The listing builds one solid part. Answer for the finished solid, in the listing's coordinates (mm). Coordinates: 2 decimals unless noted, no trailing zeros. Loops run counter-clockwise (first coordinate to the right, second up) from the corner with the lowest first, then second, coordinate; pieces in that order, holes last. Notation, with made-up numbers: M 7,12 L 32,12 A28 cw 32,45 Z; hole C -1.5,40.25 d4. An arc over 180 degrees is marked long. Return JSON: item names as keys, results as strings. Group by question number.
1. Section A-A (z = -56.5) is taken. Write down the section's boundary in (x, y), then the cut area to 3 significant figures.
2. Section D-D (x = 64) is taken. Write down the section's boundary in (y, z).
3. Section B-B (y = 0.7) is taken. Count the separate pieces of the cut face and the enclosed holes in it, then the cut area to 3 significant figures.
4. Section C-C (z = 13) is taken. Write down the section's boundary in (x, y), then the cut area to 3 significant figures.
5. Given P1, Ø1.3, axis at y = 1, z = 66, coming from the +X side; P2, Ø1.2, axis at y = 1.5, z = 69, coming from the +X side; P3, Ø1.2, axis at y = 1, z = 69, coming from the -X side, each flat-ended and moving along its own axis, determine where each tip first touches the part or whether it passes through.
6. Straight lines are drawn through the part: L1, parallel to X at y = 2.4, z = -7; L2, parallel to X at y = 2.9, z = -66.5; L3, parallel to Z at x = -30, y = 2.5. For each, find the intervals that lie inside material, in ascending order. Write a range as from..to.
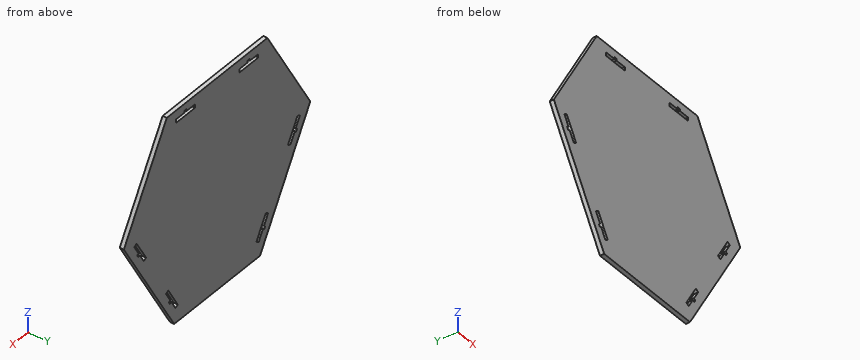
```python
from build123d import *

# Parameters (mm, degrees)
BOSS_EXTRUDE1_DEPTH      = 3
CUT_EXTRUDE1_DEPTH       = 119.131597452
CIRPATTERN1_COUNT        = 3
CIRPATTERN1_COPY_1_DEPTH = 119.131597452
CIRPATTERN1_COPY_2_DEPTH = 119.131597452


with BuildPart() as part:
    # Sketch1 → Boss-Extrude1 (new body)
    with BuildSketch(Plane(origin=(0, 0, 0), x_dir=(1, 0, 0), z_dir=(0, 1, 0))):
        Polygon((-40.640000094, 78.456128134), (40.639999906, 78.456128134), (88.265000282, -4.032791576), (47.624999812, -74.423336558), (-47.625, -74.423336558), (-88.265000094, -4.032791576), align=None)
    extrude(amount=BOSS_EXTRUDE1_DEPTH)

    # Sketch2 → Cut-Extrude1 (cut, through all)
    with BuildSketch(Plane(origin=(0, 3, 0), x_dir=(1, 0, 0), z_dir=(0, 1, 0))):
        Polygon((29, -68), (29, -69.5), (31, -69.5), (31, -68), (38.96, -68), (38.96, -65.48), (21.04, -65.48), (21.04, -68), align=None)
    cut_extrude1 = extrude(amount=-CUT_EXTRUDE1_DEPTH, mode=Mode.SUBTRACT)

    # Mirror1: Cut-Extrude1 across plane
    add(cut_extrude1.mirror(Plane(origin=(0, 0, 0), x_dir=(0, 0, 1), z_dir=(1, 0, 0))), mode=Mode.SUBTRACT)

    # CirPattern1: Cut-Extrude1 ×3 about axis
    cirpattern1_axis = Axis((0, 0, 0), (0, 1, 0))
    for i in range(1, CIRPATTERN1_COUNT):
        add(cut_extrude1.rotate(cirpattern1_axis, i * 360 / CIRPATTERN1_COUNT), mode=Mode.SUBTRACT)

    # CirPattern1 copy 1 sketch → CirPattern1 copy 1 (cut, through all)
    with BuildSketch(Plane(origin=(0, 3, 0), x_dir=(0.4999999999999998, 0, 0.8660254037844387), z_dir=(0, 1, 0))):
        Polygon((29, 68), (29, 69.5), (31, 69.5), (31, 68), (38.96, 68), (38.96, 65.48), (21.04, 65.48), (21.04, 68), align=None)
    extrude(amount=-CIRPATTERN1_COPY_1_DEPTH, mode=Mode.SUBTRACT)

    # CirPattern1 copy 2 sketch → CirPattern1 copy 2 (cut, through all)
    with BuildSketch(Plane(origin=(0, 3, 0), x_dir=(0.5000000000000004, 0, -0.8660254037844384), z_dir=(0, 1, 0))):
        Polygon((29, 68), (29, 69.5), (31, 69.5), (31, 68), (38.96, 68), (38.96, 65.48), (21.04, 65.48), (21.04, 68), align=None)
    extrude(amount=-CIRPATTERN1_COPY_2_DEPTH, mode=Mode.SUBTRACT)


solid = part.part
```
Worked out:
{
 "1": {"outline": "M -53.32,0 L -45.9,0 L -45.9,3 L -53.32,3 Z; M -42.99,0 L 42.99,0 L 42.99,3 L -42.99,3 Z; M 45.9,0 L 53.32,0 L 53.32,3 L 45.9,3 Z", "area": "302 mm^2"},
 "2": {"outline": "M 0,-38 L 3,-38 L 3,46.06 L 0,46.06 Z"},
 "3": {"separate pieces": "1", "enclosed holes": "6", "area": "19,900 mm^2"},
 "4": {"outline": "M -83.09,0 L 83.09,0 L 83.09,3 L -83.09,3 Z", "area": "499 mm^2"},
 "5": {"P1": "x = 52.86", "P2": "x = 51.1", "P3": "x = -51.1"},
 "6": {"L1": "-81.9..-74.48, -71.57..71.57, 74.48..81.9", "L2": "-47.54..-40.13, -37.26..37.26, 40.13..47.54", "L3": "-78.46..65.48, 69.5..74.42"}
}
